Solid Edge part; units mm, degrees
sketch "Sketch1" plane through (0, 0, 0) normal (0, 0, 1) x (1, 0, 0)
  circle A0 centre (-54.7801, 10.6787) radius 75
extrude "Protrusion1" add sketch "Sketch1" along normal blind 50
hole "Hole_1" at (-54.7801, 10.6787, 50) direction (0, 0, -1) diameter 100 end up to next
sketch "Sketch2" plane through (-54.7801, 10.6787, 50) normal (0, 0, 1) x (1, 0, 0)
  arc A0 (60, 0) -> (42.4264, 42.4264) centre (0, 0) ccw
  line L0 (56.5685, 56.5685) -> (42.4264, 42.4264)
  arc A1 (80, 0) -> (56.5685, 56.5685) centre (0, 0) ccw
  line L1 (60, 0) -> (80, 0)
extrude "Cutout1" cut sketch "Sketch2" against normal through all
pattern_circular "Pattern1" count 2 over 360 about axis through (-54.7801, 10.6787, 50) along (0, 0, -1) of "Cutout1"
For this review, take the finished solid that the model builds, in its own axes (mm). A direction names the side the tool comes from. Give positions to 0.01 mm unless a question says otherwise; leave off trailing zeros. Write each loop counter-clockwise with the first axis right and the second up, starting at its lowest first coordinate (ties: lowest second). Pieces come first, ordered by that corner, then holes. Notation, with made-up numbers: (50, 68.25) -> (106, 68.25) arc R15 cw to (106, 94.25) -> close; hole circle Ø11 at (39, 73.25). An arc over 180 degrees is marked (long way). Use CSV: the item, a comma, the result in double quotes.
Q1. Take a section at C-C, the plane z = 22. Write out the cut boundary in (x, y), then the cut area to 3 significant figures.
Conclusion:
outline,"(-129.78, 10.68) -> (-114.78, 10.68) arc R60 ccw to (-97.21, -31.75) -> (-107.81, -42.35) arc R75 ccw to (20.22, 10.68) -> (5.22, 10.68) arc R60 ccw to (-12.35, 53.11) -> (-1.75, 63.71) arc R75 ccw to start; hole circle Ø100 at (-54.78, 10.68)"
area,"8,230 mm2"
Q2. To check wall thickness, follow probe 1 along X at (y, z) = (-13.5, 48); probe 2 along Y at (x, z) = (-105, 37); probe 3 along Y at (x, z) = (-42, 33). State the ranges of each line that lie inside material, in increasing order. Write a range as [from, to].
Conclusion:
probe 1,"[-109.69, -98.55], [-11.01, 16.22]"
probe 2,"[-45.03, -39.54], [-22.15, 66.38]"
probe 3,"[-63.22, -37.66], [59.02, 84.58]"
Q3. Take a section at D-D, the plane x = -120. Write out the cut boundary in (y, z), then the cut area to 3 significant figures.
Conclusion:
outline,"(10.68, 0) -> (47.71, 0) -> (47.71, 50) -> (10.68, 50) -> close"
area,"1,850 mm2"
Q4. Tool access review of faces 4 (the face through (-6.98, 58.48, 25.35)), 5 (the face through (13, 10.679, 25)), 6 (the face through (-102.584, -37.125, 25.35)), 7 (the face through (-6, -5, 0)), 8 (the face through (-122, 10.679, 25)): name each direction out of +Z, -Z, +X, -X, +Y, -Y from which nothing blocks a thin tool from reaching the whole face with its end or side.
Conclusion:
face 4,"+Z, -Z, +X"
face 5,"+Z, -Z, +X, +Y"
face 6,"+Z, -Z, -X"
face 7,"-Z, +X, -X, +Y, -Y"
face 8,"+Z, -Z, -X, -Y"
Q5. Take a section at B-B, the plane x = -85. Write out the cut boundary in (y, z).
Conclusion:
outline,"(-57.96, 0) -> (-29.16, 0) -> (-29.16, 50) -> (-57.96, 50) -> close; (50.51, 0) -> (79.32, 0) -> (79.32, 50) -> (50.51, 50) -> close"
Q6. For P1, Ø7.5, axis at x = 13, z = 22.5, coming from the +Y side; P2, Ø7.5, axis at x = -123.5, z = 34.5, coming from the -Y side; P3, Ø10, axis at y = 52.5, z = 30.5, coming from the -X side, all flat-tipped, find the tip position at first contact; note any pin that passes through.
Conclusion:
P1,"y = 10.68"
P2,"y = 10.68"
P3,"x = -120.12"
Q7. Mouldability with a two-part tool opening along X and no side actions: class faces 1 (the face through (-24.94, -58.13, 24.65)), 2 (the face through (-6, -5, 50)), 3 (the face through (-99.14, -12.39, 25.35)) as pulls with the +X half, pulls with the -X half, needs draft (parallel to the pull), parting line crosses it, or undercut.
Conclusion:
face 1,"parting line crosses it"
face 2,"needs draft"
face 3,"undercut"
Q8. Take a section at A-A, the plane y = 34. Write out the cut boundary in (x, z), then the cut area to 3 significant figures.
Conclusion:
outline,"(-126.06, 0) -> (-99.01, 0) -> (-99.01, 50) -> (-126.06, 50) -> close; (-10.55, 0) -> (0.5, 0) -> (0.5, 50) -> (-10.55, 50) -> close"
area,"1,910 mm2"
